Part model, mm, in its own coordinate system. A direction names the side the tool comes from. Give positions to 0.01 mm unless a question says otherwise; leave off trailing zeros. Write each loop counter-clockwise with the first axis right and the second up, starting at its lowest first coordinate (ties: lowest second). Pieces come first, ordered by that corner, then holes. Notation, with made-up numbers: M 45.25,-14.75 L 82.25,-14.75 A21 ccw 82.25,-9.75 Z; hole C 14,17.25 d8. An arc over 180 degrees is marked long. Answer as CSV lines item,"result". Start each with the question number.
1) Slice it at A-A, the plane z = -10.5. Give the cut face in (x, y), plus the area to 3 significant figures.
2) Pin check, flat tips, straight feed: pin 1 Ø5 at (x, y) = (3, 26.5) entering from -Z; pin 2 Ø7.5 at (x, z) = (18.19, -10.5) entering from +Y; pin 3 Ø6 at (x, y) = (14, 20.5) entering from +Z. Stop position of each tip, or through.
3) Tool access for faces 4 (the flat face through (20, 25, 35)), 5 (the cylindrical face through (15.791, 8.521, 8.303)), 6 (the flat face through (45, 35, 12)): list every direction of +Z, -Z, +X, -X, +Y, -Y with a clear straight run to the whole face (end or side of a thin tool).
4) Wall check: line 1 along Y through (x, z) = (10, 34); line 2 along X through (y, z) = (4, -10.5); line 3 along X through (y, z) = (30, 79.5). Give the ranges that are in metal, low to high. Write a range as from..to.
5) Slice it at C-C, the plane z = -43. Give the cut face in (x, y).
6) Slice it at B-B, the plane z = 41.5. Give the cut face in (x, y), plus the area to 3 significant figures.
7) Slice it at D-D, the plane x = -11. Give the cut face in (y, z).
8) Mould opens along Y. For faces 1 (the cylindrical face through (-44.54, 27.39, 73.94)), 2 (the flat face through (0, 9, -60)), 3 (the cylindrical face through (-45, 34, -58)) say: pulls with the +Y half, pulls with the -Y half, needs draft (parallel to the pull), parting line crosses it, or undercut.
```python
from build123d import *

# Parameters (mm, degrees)
BOSS_EXTRUDE1_DEPTH            = 85
BOSS_EXTRUDE1_DEPTH_BACK       = 60
SKETCH4_R                      = 7.5
CUT_EXTRUDE1_DEPTH             = 80
CBORE_FOR_M3_SHCS1_D           = 3.5
CBORE_FOR_M3_SHCS1_CBORE_D     = 6.5
CBORE_FOR_M3_SHCS1_CBORE_DEPTH = 3
CIRPATTERN1_COUNT              = 6
SKETCH5_R                      = 1.75
CUT_EXTRUDE2_DEPTH             = 132.476233594
LPATTERN1_COUNT                = 6
LPATTERN1_PITCH                = 25
SKETCH6_R                      = 1.75
CUT_EXTRUDE3_DEPTH             = 101.294566154
FILLET1_R                      = 5
FILLET2_R                      = 3
SKETCH9_R                      = 1.75
CUT_EXTRUDE6_DEPTH             = 10
SKETCH10_R                     = 3
CUT_EXTRUDE7_DEPTH             = 1.5
SKETCH11_W                     = 20
SKETCH11_H                     = 20
BOSS_EXTRUDE2_DEPTH            = 27
SKETCH12_R                     = 1.75
CUT_EXTRUDE8_DEPTH             = 104.937481209
CHAMFER1_SIZE                  = 4


with BuildPart() as part:
    # Sketch1 → Boss-Extrude1 (new, two sides: drawn at the far end of the back side and taken through both)
    with BuildSketch(Plane.XY.offset(-BOSS_EXTRUDE1_DEPTH_BACK)):
        Polygon((-47, 35), (-47, 0), (47, 0), (47, 35), (42, 35), (42, 10), (-42, 10), (-42, 35), align=None)
    extrude(amount=BOSS_EXTRUDE1_DEPTH + BOSS_EXTRUDE1_DEPTH_BACK)

    # Sketch4 → Cut-Extrude1 (cut)
    with BuildSketch(Plane(origin=(0, 10, 0), x_dir=(1, 0, 0), z_dir=(0, 1, 0))):
        with Locations(Location((0, 0, 0), (0, 0, 270))):
            Circle(SKETCH4_R)
    extrude(amount=-CUT_EXTRUDE1_DEPTH, mode=Mode.SUBTRACT)

    # CBORE for M3 SHCS1 (through all)
    with Locations(Plane(origin=(0, 10, 0), x_dir=(1, 0, 0), z_dir=(0, 1, 0))):
        with Locations((0, 21)):
            cbore_for_m3_shcs1 = CounterBoreHole(CBORE_FOR_M3_SHCS1_D / 2, CBORE_FOR_M3_SHCS1_CBORE_D / 2, CBORE_FOR_M3_SHCS1_CBORE_DEPTH)

    # CirPattern1: CBORE for M3 SHCS1 ×6 about axis
    cirpattern1_axis = Axis((0, 0, 0), (0, 1, 0))
    for i in range(1, CIRPATTERN1_COUNT):
        add(cbore_for_m3_shcs1.rotate(cirpattern1_axis, i * 360 / CIRPATTERN1_COUNT), mode=Mode.SUBTRACT)

    # Sketch5 → Cut-Extrude2 (cut, through all)
    with BuildSketch(Plane.ZY.offset(47)):
        with Locations(Location((-50, 26, 0), (0, 0, 270))):
            Circle(SKETCH5_R)
    cut_extrude2 = extrude(amount=-CUT_EXTRUDE2_DEPTH, mode=Mode.SUBTRACT)

    # LPattern1: Cut-Extrude2 ×6
    with Locations(*[(0, 0, i * LPATTERN1_PITCH) for i in range(1, LPATTERN1_COUNT)]):
        add(cut_extrude2, mode=Mode.SUBTRACT)

    # Sketch6 → Cut-Extrude3 (cut, through all)
    with BuildSketch(Plane(origin=(0, 10, 0), x_dir=(1, 0, 0), z_dir=(0, 1, 0))):
        with Locations(Location((0, -59.5, 0), (0, 0, 270))):
            Circle(SKETCH6_R)
        with Locations(Location((7.5, -67, 0), (0, 0, 270))):
            Circle(SKETCH6_R)
        with Locations(Location((0, -74.5, 0), (0, 0, 270))):
            Circle(SKETCH6_R)
        with Locations(Location((-7.5, -67, 0), (0, 0, 270))):
            Circle(SKETCH6_R)
    extrude(amount=-CUT_EXTRUDE3_DEPTH, mode=Mode.SUBTRACT)

    # Fillet1
    fillet1_edges = [part.edges().sort_by_distance(p)[0] for p in [
        (0, 0, -60),
        (44.5, 35, -60),
        (-44.5, 35, 85),
        (0, 0, 85),
        (44.5, 35, 85),
        (-44.5, 35, -60),
    ]]
    fillet(fillet1_edges, radius=FILLET1_R)

    # Fillet2
    fillet2_edges = [part.edges().sort_by_distance(p)[0] for p in [
        (-42, 10, 12.5),
        (42, 10, 12.5),
    ]]
    fillet(fillet2_edges, radius=FILLET2_R)

    # Sketch9 → Cut-Extrude6 (cut)
    with BuildSketch(Plane(origin=(47, 0, 0), x_dir=(0, 0, -1), z_dir=(1, 0, 0))):
        with Locations(Location((0, 16, 0), (0, 0, 90))):
            Circle(SKETCH9_R)
    extrude(amount=-CUT_EXTRUDE6_DEPTH, mode=Mode.SUBTRACT)

    # Sketch10 → Cut-Extrude7 (cut)
    with BuildSketch(Plane.ZY.offset(-42)):
        with Locations((0, 16)):
            Circle(SKETCH10_R)
    extrude(amount=-CUT_EXTRUDE7_DEPTH, mode=Mode.SUBTRACT)

    # Sketch11 → Boss-Extrude2 (add)
    with BuildSketch(Plane(origin=(0, 10, 0), x_dir=(1, 0, 0), z_dir=(0, 1, 0))):
        with Locations((10, -35)):
            Rectangle(SKETCH11_W, SKETCH11_H)
    extrude(amount=BOSS_EXTRUDE2_DEPTH)

    # Sketch12 → Cut-Extrude8 (cut, through all)
    with BuildSketch(Plane.XY):
        with Locations(Location((10, 25, 0), (0, 0, 180))):
            Circle(SKETCH12_R)
        with Locations(Location((10, 33.5, 0), (0, 0, 180))):
            Circle(SKETCH12_R)
    extrude(amount=CUT_EXTRUDE8_DEPTH, mode=Mode.SUBTRACT)

    # Chamfer1
    # the kernel refuses this chamfer: 4 mm, written as the material it adds along each edge
    with BuildSketch(Plane(origin=(0, 10, 45), x_dir=(0, -0.02749587661058651, 0.9996219169112968), z_dir=(1, 0, 0)), Plane(origin=(20, 10, 45), x_dir=(0.9996219169112968, -0.027495876610586487, 0), z_dir=(0, 0, -1)), Plane(origin=(0, 10, 25), x_dir=(-0.9996219169112968, -0.02749587661058648, 0), z_dir=(0, 0, 1))) as chamfer1_piece_1:
        Polygon((CHAMFER1_SIZE * 0.999621916911, -CHAMFER1_SIZE * 0.0274958766106), (-CHAMFER1_SIZE * 0.0274958766106, -CHAMFER1_SIZE * 0.999621916911), (0, 0), align=None)
    extrude(amount=20)
    with BuildSketch(Plane(origin=(20, 10, 25), x_dir=(0, -0.027495876610586487, -0.9996219169112968), z_dir=(-1, 0, 0))) as chamfer1_piece_2_section:
        Polygon((CHAMFER1_SIZE * 0.999621916911, -CHAMFER1_SIZE * 0.0274958766106), (-CHAMFER1_SIZE * 0.0274958766106, -CHAMFER1_SIZE * 0.999621916911), (0, 0), align=None)
    chamfer1_piece_2 = extrude(amount=20, mode=Mode.PRIVATE)
    chamfer1_piece_2 = chamfer1_piece_2 - Plane(origin=(0, 11.352573601, 21), x_dir=(-1, 0, 0), z_dir=(0, 1, 0)) * Cylinder(3.25, 56, mode=Mode.PRIVATE)
    add(chamfer1_piece_2)
    with BuildSketch(Plane(origin=(0, 10, 25), x_dir=(-0.9996219169112968, -0.02749587661058648, 0), z_dir=(0, 0, 1))) as chamfer1_piece_3a_section:
        Polygon((CHAMFER1_SIZE * 0.999621916911, -CHAMFER1_SIZE * 0.0274958766106), (-CHAMFER1_SIZE * 0.0274958766106, -CHAMFER1_SIZE * 0.999621916911), (0, 0), align=None)
    chamfer1_piece_3a = extrude(amount=30.286731952, mode=Mode.PRIVATE)
    chamfer1_piece_3a = split(chamfer1_piece_3a, bisect_by=Plane(origin=(-1.319174507, 11.319174507, 45), z_dir=(0, 0, 1)), keep=Keep.TOP, mode=Mode.PRIVATE)
    with BuildSketch(Plane(origin=(-10.286731952, 10, 45), x_dir=(0, -0.02749587661058651, 0.9996219169112968), z_dir=(1, 0, 0))) as chamfer1_piece_3b_section:
        Polygon((CHAMFER1_SIZE * 0.999621916911, -CHAMFER1_SIZE * 0.0274958766106), (-CHAMFER1_SIZE * 0.0274958766106, -CHAMFER1_SIZE * 0.999621916911), (0, 0), align=None)
    chamfer1_piece_3b = extrude(amount=30.286731952, mode=Mode.PRIVATE)
    chamfer1_piece_3b = split(chamfer1_piece_3b, bisect_by=Plane(origin=(0, 11.319174507, 46.319174507), z_dir=(-1, 0, 0)), keep=Keep.TOP, mode=Mode.PRIVATE)
    chamfer1_piece_3 = chamfer1_piece_3a & chamfer1_piece_3b
    add(chamfer1_piece_3)
    with BuildSketch(Plane(origin=(20, 10, 55.286731952), x_dir=(0.9996219169112968, -0.027495876610586487, 0), z_dir=(0, 0, -1))) as chamfer1_piece_4a_section:
        Polygon((CHAMFER1_SIZE * 0.999621916911, -CHAMFER1_SIZE * 0.0274958766106), (-CHAMFER1_SIZE * 0.0274958766106, -CHAMFER1_SIZE * 0.999621916911), (0, 0), align=None)
    chamfer1_piece_4a = extrude(amount=30.286731952, mode=Mode.PRIVATE)
    chamfer1_piece_4a = split(chamfer1_piece_4a, bisect_by=Plane(origin=(21.319174507, 11.319174507, 45), z_dir=(0, 0, 1)), keep=Keep.TOP, mode=Mode.PRIVATE)
    with BuildSketch(Plane(origin=(0, 10, 45), x_dir=(0, -0.02749587661058651, 0.9996219169112968), z_dir=(1, 0, 0))) as chamfer1_piece_4b_section:
        Polygon((CHAMFER1_SIZE * 0.999621916911, -CHAMFER1_SIZE * 0.0274958766106), (-CHAMFER1_SIZE * 0.0274958766106, -CHAMFER1_SIZE * 0.999621916911), (0, 0), align=None)
    chamfer1_piece_4b = extrude(amount=30.286731952, mode=Mode.PRIVATE)
    chamfer1_piece_4b = split(chamfer1_piece_4b, bisect_by=Plane(origin=(20, 11.319174507, 46.319174507), z_dir=(1, 0, 0)), keep=Keep.TOP, mode=Mode.PRIVATE)
    chamfer1_piece_4 = chamfer1_piece_4a & chamfer1_piece_4b
    add(chamfer1_piece_4)
    with BuildSketch(Plane(origin=(30.286731952, 10, 25), x_dir=(0, -0.027495876610586487, -0.9996219169112968), z_dir=(-1, 0, 0))) as chamfer1_piece_5a_section:
        Polygon((CHAMFER1_SIZE * 0.999621916911, -CHAMFER1_SIZE * 0.0274958766106), (-CHAMFER1_SIZE * 0.0274958766106, -CHAMFER1_SIZE * 0.999621916911), (0, 0), align=None)
    chamfer1_piece_5a = extrude(amount=30.286731952, mode=Mode.PRIVATE)
    chamfer1_piece_5a = split(chamfer1_piece_5a, bisect_by=Plane(origin=(20, 11.319174507, 23.680825493), z_dir=(1, 0, 0)), keep=Keep.TOP, mode=Mode.PRIVATE)
    with BuildSketch(Plane(origin=(20, 10, 45), x_dir=(0.9996219169112968, -0.027495876610586487, 0), z_dir=(0, 0, -1))) as chamfer1_piece_5b_section:
        Polygon((CHAMFER1_SIZE * 0.999621916911, -CHAMFER1_SIZE * 0.0274958766106), (-CHAMFER1_SIZE * 0.0274958766106, -CHAMFER1_SIZE * 0.999621916911), (0, 0), align=None)
    chamfer1_piece_5b = extrude(amount=30.286731952, mode=Mode.PRIVATE)
    chamfer1_piece_5b = split(chamfer1_piece_5b, bisect_by=Plane(origin=(21.319174507, 11.319174507, 25), z_dir=(0, 0, -1)), keep=Keep.TOP, mode=Mode.PRIVATE)
    chamfer1_piece_5 = chamfer1_piece_5a & chamfer1_piece_5b
    add(chamfer1_piece_5)
    with BuildSketch(Plane(origin=(0, 10, 14.713268048), x_dir=(-0.9996219169112968, -0.027495876610586494, 0), z_dir=(0, 0, 1))) as chamfer1_piece_6a_section:
        Polygon((CHAMFER1_SIZE * 0.999621916911, -CHAMFER1_SIZE * 0.0274958766106), (-CHAMFER1_SIZE * 0.0274958766106, -CHAMFER1_SIZE * 0.999621916911), (0, 0), align=None)
    chamfer1_piece_6a = extrude(amount=30.286731952, mode=Mode.PRIVATE)
    chamfer1_piece_6a = chamfer1_piece_6a - Plane(origin=(0, 10.566435826, 21), x_dir=(-1, 0, 0), z_dir=(0, 1, 0)) * Cylinder(3.25, 77, mode=Mode.PRIVATE)
    chamfer1_piece_6a = split(chamfer1_piece_6a, bisect_by=Plane(origin=(-3.383951939, 10.566435826, 25), z_dir=(0, 0, -1)), keep=Keep.TOP, mode=Mode.PRIVATE)
    with BuildSketch(Plane(origin=(20, 10, 25), x_dir=(0, -0.027495876610586487, -0.9996219169112968), z_dir=(-1, 0, 0))) as chamfer1_piece_6b_section:
        Polygon((CHAMFER1_SIZE * 0.999621916911, -CHAMFER1_SIZE * 0.0274958766106), (-CHAMFER1_SIZE * 0.0274958766106, -CHAMFER1_SIZE * 0.999621916911), (0, 0), align=None)
    chamfer1_piece_6b = extrude(amount=30.286731952, mode=Mode.PRIVATE)
    chamfer1_piece_6b = chamfer1_piece_6b - Plane(origin=(0, 11.389114273, 21), x_dir=(-1, 0, 0), z_dir=(0, 1, 0)) * Cylinder(3.25, 77, mode=Mode.PRIVATE)
    chamfer1_piece_6b = split(chamfer1_piece_6b, bisect_by=Plane(origin=(0, 11.389114273, 23.812991609), z_dir=(-1, 0, 0)), keep=Keep.TOP, mode=Mode.PRIVATE)
    chamfer1_piece_6 = chamfer1_piece_6a & chamfer1_piece_6b
    add(chamfer1_piece_6)


solid = part.part
```
Found:
1,outline,"M -47,0 L -19.94,0 L -19.94,7 L -21.44,7 L -21.44,10 L -39,10 A3 cw -42,13 L -42,35 L -47,35 Z; M -16.44,0 L 16.44,0 L 16.44,7 L 14.94,7 L 14.94,10 L -14.94,10 L -14.94,7 L -16.44,7 Z; M 19.94,0 L 47,0 L 47,35 L 42,35 L 42,13 A3 cw 39,10 L 21.44,10 L 21.44,7 L 19.94,7 Z"
1,area,"1,110 mm²"
2,pin 1,"z = 25"
2,pin 2,"y = 10"
2,pin 3,"z = 45"
3,face 4,"+Z, -Z, +Y"
3,face 5,"+Y"
3,face 6,"+Z, -Z, +X, +Y"
4,line 1,"0..23.25, 26.75..31.75, 35.25..37"
4,line 2,"-47..-19.94, -16.44..16.44, 19.94..47"
4,line 3,"-47..-42, 42..47"
5,outline,"M -47,0 L 47,0 L 47,35 L 42,35 L 42,13 A3 cw 39,10 L -39,10 A3 cw -42,13 L -42,35 L -47,35 Z"
6,outline,"M -47,0 L 47,0 L 47,35 L 42,35 L 42,13 A3 cw 39,10 L 24,10 L 20,14 L 20,37 L 0,37 L 0,14 L -4,10 L -39,10 A3 cw -42,13 L -42,35 L -47,35 Z; hole C 10,25 d3.5; hole C 10,33.5 d3.5"
6,area,"1,730 mm²"
7,outline,"M 0,-55 A5 ccw 5,-60 L 10,-60 L 10,85 L 5,85 A5 ccw 0,80 Z"
8,face 1,"undercut"
8,face 2,"needs draft"
8,face 3,"pulls with the +Y half"
